The listing builds one solid part. Answer for the finished solid, in the listing's coordinates (mm). Face numbers are marked on the shaded views. A direction names the side the tool comes from. Coordinates: 2 decimals unless noted, no trailing zeros. Write each loop counter-clockwise with the first axis right and the second up, starting at its lowest first coordinate (ties: lowest second). Pieces come first, ordered by that corner, then holes.
from build123d import *

# Parameters (mm, degrees)
F0_W      = 53
F0_H      = 53
F1_DEPTH  = 10
F2_W      = 43
F2_H      = 43
F3_DEPTH  = 5
F4_R      = 1.7
F5_DEPTH  = 25
F6_R      = 11.2
F7_DEPTH  = 25
F9_DEPTH  = 48
F10_DEPTH = 29
F11_R     = 15
F12_DEPTH = 53.001
F13_R     = 12.5
F14_DEPTH = 53.001
F15_W     = 5
F15_H     = 58
F16_DEPTH = 25
F17_SIZE2 = 53
F17_SIZE  = 25
F18_W     = 43
F18_H     = 5
F19_DEPTH = 25
F20_R     = 5
F21_DEPTH = 25
F22_W     = 15
F22_H     = 5
F23_DEPTH = 15
F24_R     = 5
F25_R     = 4
F26_DEPTH = 25


# Not quite as in the source:
# - a pattern or mirror of a feature is missing from the dataset's text; its kind, count and spacing are read off the source's solid


with BuildPart() as f1:
    # F0 (on Top) → F1 (new body)
    with BuildSketch(Plane.XY):
        Rectangle(F0_W, F0_H)
    extrude(amount=F1_DEPTH)

    # F2 (on face) → F3 (cut)
    with BuildSketch(Plane.XY.offset(10)):
        Rectangle(F2_W, F2_H)
    extrude(amount=-F3_DEPTH, mode=Mode.SUBTRACT)

    # F4 (on face) → F5 (cut)
    with BuildSketch(Plane(origin=(0, 0, 0), x_dir=(1, 0, 0), z_dir=(0, 0, -1))):
        with Locations((-16.5182938799, 16.5182938799)):
            Circle(F4_R)
        with Locations((16.0086180547, 16.5182938799)):
            Circle(F4_R)
        with Locations((16.0086180547, -16.0086180547)):
            Circle(F4_R)
        with Locations((-16.5182938799, -16.0086180547)):
            Circle(F4_R)
    extrude(amount=-F5_DEPTH, mode=Mode.SUBTRACT)

    # F6 (on face) → F7 (cut)
    with BuildSketch(Plane(origin=(0, 0, 0), x_dir=(1, 0, 0), z_dir=(0, 0, -1))):
        Circle(F6_R)
    extrude(amount=-F7_DEPTH, mode=Mode.SUBTRACT)

    # F8 (on face) → F9 (join)
    with BuildSketch(Plane.XY.offset(10)):
        Polygon((-21.5, -21.5), (-21.5, 21.5), (-21.5, 26.5), (-26.5, 26.5), (-26.5, -26.5), (-21.5, -26.5), align=None)
        Polygon((21.5, 26.5), (21.5, 21.5), (21.5, -21.5), (21.5, -26.5), (26.5, -26.5), (26.5, 26.5), align=None)
    extrude(amount=F9_DEPTH)

    # F10 (add): faces of the model
    f10_faces = [f1.faces().sort_by_distance(p)[0] for p in [
        (0, 24, 10),
        (0, -24, 10),
    ]]
    extrude(f10_faces, amount=F10_DEPTH)

    # F11 (on face) → F12 (cut, through all)
    with BuildSketch(Plane.YZ.offset(26.5)):
        with Locations((0, 30.6356716901)):
            Circle(F11_R)
    extrude(amount=-F12_DEPTH, mode=Mode.SUBTRACT)

    # F13 (on face) → F14 (cut, through all)
    with BuildSketch(Plane(origin=(0, 26.5, 0), x_dir=(-1, 0, 0), z_dir=(0, 1, 0))):
        with Locations((0, 19.5)):
            Circle(F13_R)
    extrude(amount=-F14_DEPTH, mode=Mode.SUBTRACT)

    # F15 (on face) → F16 (join)
    with BuildSketch(Plane(origin=(-26.5, 0, 0), x_dir=(0, -1, 0), z_dir=(-1, 0, 0))):
        with Locations((-24, 29)):
            Rectangle(F15_W, F15_H)
        with Locations((24, 29)):
            Rectangle(F15_W, F15_H)
    f16 = extrude(amount=F16_DEPTH)

    # F16_copies: F16 across plane
    add(f16.mirror(Plane(origin=(0, 0, 0), x_dir=(0, 0, 1), z_dir=(1, 0, 0))))

    # F17
    f17_edges = [f1.edges().sort_by_distance(p)[0] for p in [
        (-51.5, 24, 0),
        (-51.5, -24, 0),
        (51.5, 24, 0),
        (51.5, -24, 0),
    ]]
    f17_side = f1.faces().sort_by_distance((25.341639, 0, 0))[0]
    chamfer(f17_edges, length=F17_SIZE, length2=F17_SIZE2, reference=f17_side)

    # F18 (on face) → F19 (join)
    with BuildSketch(Plane(origin=(-26.5, 0, 0), x_dir=(0, -1, 0), z_dir=(-1, 0, 0))):
        with Locations((0, 55.5)):
            Rectangle(F18_W, F18_H)
    f19 = extrude(amount=F19_DEPTH)

    # F19_copies: F19 across plane
    add(f19.mirror(Plane(origin=(0, 0, 0), x_dir=(0, 0, 1), z_dir=(1, 0, 0))))

    # F20 (on face) → F21 (cut)
    with BuildSketch(Plane(origin=(0, 0, 53), x_dir=(1, 0, 0), z_dir=(0, 0, -1))):
        with Locations((-39, 11.5)):
            Circle(F20_R)
        with Locations((-39, -11.5)):
            Circle(F20_R)
    f21 = extrude(amount=-F21_DEPTH, mode=Mode.SUBTRACT)

    # F21_copies: F21 across plane
    add(f21.mirror(Plane(origin=(0, 0, 0), x_dir=(0, 0, 1), z_dir=(1, 0, 0))), mode=Mode.SUBTRACT)

    # F22 (on face) → F23 (join)
    with BuildSketch(Plane(origin=(0, 26.5, 0), x_dir=(-1, 0, 0), z_dir=(0, 1, 0))):
        with Locations((-19, 2.5)):
            Rectangle(F22_W, F22_H)
    f23 = extrude(amount=F23_DEPTH)

    # F23_copies: F23 across plane
    add(f23.mirror(Plane(origin=(0, 0, 0), x_dir=(0, 0, -1), z_dir=(-1, 0, 0))))

    # F24
    f24_edges = [f1.edges().sort_by_distance(p)[0] for p in [
        (11.5, 41.5, 2.5),
        (26.5, 41.5, 2.5),
        (-11.5, 41.5, 2.5),
        (-26.5, 41.5, 2.5),
    ]]
    fillet(f24_edges, radius=F24_R)

    # F25 (on face) → F26 (cut)
    with BuildSketch(Plane(origin=(0, 0, 0), x_dir=(1, 0, 0), z_dir=(0, 0, -1))):
        with Locations((19, -35.5)):
            Circle(F25_R)
    f26 = extrude(amount=-F26_DEPTH, mode=Mode.SUBTRACT)

    # F26_copies: F26 across plane
    add(f26.mirror(Plane(origin=(0, 0, 0), x_dir=(0, 0, -1), z_dir=(-1, 0, 0))), mode=Mode.SUBTRACT)


solid = f1.part
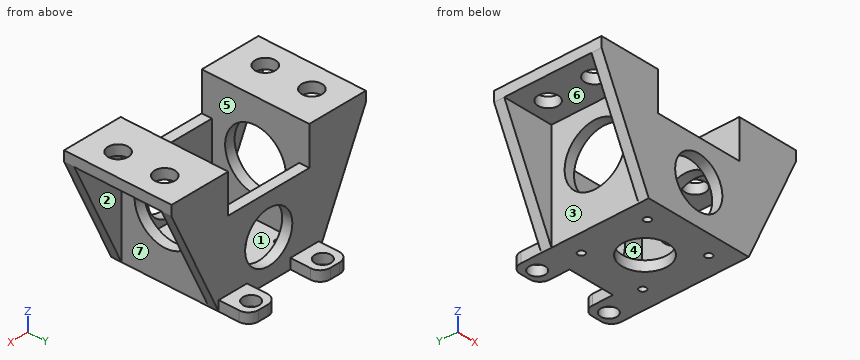
1. Section A-A on y = 0 is taken. Give the vertices of the cut face in (x, z), then the cut area to 3 significant figures.
Results found:
outline: (-51.5, 53) - (-26.5, 53) - (-26.5, 45.64) - (-21.5, 45.64) - (-21.5, 58) - (-51.5, 58) - close; (-26.5, 0) - (-11.2, 0) - (-11.2, 5) - (-21.5, 5) - (-21.5, 15.64) - (-26.5, 15.64) - close; (11.2, 0) - (26.5, 0) - (26.5, 15.64) - (21.5, 15.64) - (21.5, 5) - (11.2, 5) - close; (21.5, 45.64) - (26.5, 45.64) - (26.5, 53) - (51.5, 53) - (51.5, 58) - (21.5, 58) - close
area: 633 mm2
2. Section C-C on z = 12.5 is taken. Give the vertices of the cut face in (x, y), then the cut area to 3 significant figures.
Results found:
outline: (-32.4, -26.5) - (-10.36, -26.5) - (-10.36, -21.5) - (-21.5, -21.5) - (-21.5, 21.5) - (-10.36, 21.5) - (-10.36, 26.5) - (-32.4, 26.5) - (-32.4, 21.5) - (-26.5, 21.5) - (-26.5, -21.5) - (-32.4, -21.5) - close; (10.36, -26.5) - (32.4, -26.5) - (32.4, -21.5) - (26.5, -21.5) - (26.5, 21.5) - (32.4, 21.5) - (32.4, 26.5) - (10.36, 26.5) - (10.36, 21.5) - (21.5, 21.5) - (21.5, -21.5) - (10.36, -21.5) - close
area: 871 mm2
3. Section B-B on x = 42 is taken. Give the vertices of the cut face in (y, z), then the cut area to 3 significant figures.
Results found:
outline: (-26.5, 32.86) - (-21.5, 32.86) - (-21.5, 53) - (-15.5, 53) - (-15.5, 58) - (-26.5, 58) - close; (-7.5, 53) - (7.5, 53) - (7.5, 58) - (-7.5, 58) - close; (15.5, 53) - (21.5, 53) - (21.5, 32.86) - (26.5, 32.86) - (26.5, 58) - (15.5, 58) - close
area: 386 mm2
4. A tool of negligible diameter and unlimited length cuts with its end or side. For the marked faces 1, 2 and 3, from which of +Z, -Z, +X, -X, +Y, -Y can it reach the whole face along a straight path? Write none if from no direction.
Results found:
face 1: +Z
face 2: -Z, +X
face 3: -Z, -X
5. Find the intervals of material crossed by L1, parallel to Y at x = 39, z = 54.65; L2, parallel to Y at x = -27, z = 21, in increasing order.
Results found:
L1: y = -26.5 to -16.5, -6.5 to 6.5, 16.5 to 26.5
L2: y = -26.5 to -21.5, 21.5 to 26.5
6. Flat-ended cylindrical pins translate along their axes: P1, Ø5, axis at x = 19, y = 35.5, coming from the +Z side; P2, Ø4.5, axis at x = -19.5, y = 32.5, coming from the +Z side; P3, Ø13, axis at y = 8.5, z = 16.5, coming from the +X side; P4, Ø12.5, axis at x = 43.5, z = 22.5, coming from the +Y side. Find the tip coordinate at first contact, or state that the pin passes through.
Results found:
P1: passes through
P2: stops at z = 5
P3: stops at x = 26.5
P4: stops at y = 26.5
7. Section D-D on x = 0 is taken. Give the vertices of the cut face in (y, z).
Results found:
outline: (-26.5, 0) - (-11.2, 0) - (-11.2, 5) - (-21.5, 5) - (-21.5, 7) - (-26.5, 7) - close; (-26.5, 32) - (-21.5, 32) - (-21.5, 39) - (-26.5, 39) - close; (11.2, 0) - (26.5, 0) - (26.5, 7) - (21.5, 7) - (21.5, 5) - (11.2, 5) - close; (21.5, 32) - (26.5, 32) - (26.5, 39) - (21.5, 39) - close
8. For a pull along X with two mould halves and no side action, classify the marked faces 4, 5, 6 and 7 as pulls with the +X half, pulls with the -X half, needs draft (parallel to the pull), parting line crosses it, or undercut.
Results found:
face 4: undercut
face 5: undercut
face 6: needs draft
face 7: pulls with the +X half
